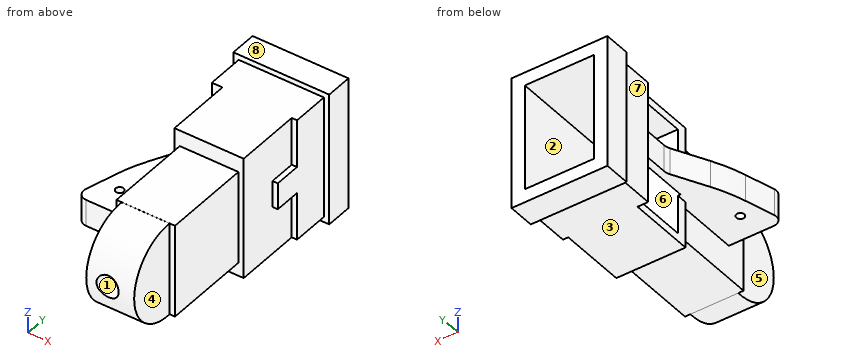
```python
from build123d import *

# Parameters (mm, degrees)
CONE002_ROLL_ANGLE   = 90
BOX005_W             = 26
BOX005_H             = 50
BOX005_DEPTH         = 40
BOX001_W             = 32
BOX001_H             = 17
BOX001_DEPTH         = 46
BOX002_W             = 26
BOX002_H             = 12
BOX002_DEPTH         = 10
BOX003_W             = 26
BOX003_H             = 26
BOX003_DEPTH         = 46
BOX004_W             = 22
BOX004_H             = 36
BOX004_DEPTH         = 35
CYLINDER_R           = 17.5
CYLINDER_DEPTH       = 18
CYLINDER_PITCH_ANGLE = 90
SKETCH001_R          = 1.5
PAD_DEPTH            = 4.5
PAD_DEPTH_BACK       = 5.5
BOX_W                = 36
BOX_H                = 10
BOX_DEPTH            = 50


with BuildPart() as obj1:
    # Cone002 → Cone002 (revolve)
    with BuildSketch(Plane.XZ):
        Polygon((0, 0), (3.9, 0), (4.2, 11), (0, 11), align=None)
    revolve(axis=Axis((0, 0, 0), (0, 0, 1)))


with BuildPart() as obj1_1:
    # Cone002 roll: moved
    add(obj1.part.rotate(Axis((0, 0, 0), (1, 0, 0)), CONE002_ROLL_ANGLE))


with BuildPart() as obj1_2:
    # Cone002 placement: moved
    add(obj1_1.part.moved(Location((32, 35, 35.5))))


with BuildPart() as kopfloch:
    # Box005 → Box005 (new body)
    with BuildSketch(Plane(origin=(19, 81, 16), x_dir=(1, 0, 0), z_dir=(0, 0, 1))):
        with Locations((13, 25)):
            Rectangle(BOX005_W, BOX005_H)
    extrude(amount=BOX005_DEPTH)


with BuildPart() as obj2:
    # Box001 → Box001 (new body)
    with BuildSketch(Plane(origin=(16, 102, 13), x_dir=(1, 0, 0), z_dir=(0, 0, 1))):
        with Locations((16, 8.5)):
            Rectangle(BOX001_W, BOX001_H)
    extrude(amount=BOX001_DEPTH)


with BuildPart() as obj3:
    # Box002 → Box002 (new body)
    with BuildSketch(Plane(origin=(22, 92, 31), x_dir=(1, 0, 0), z_dir=(0, 0, 1))):
        with Locations((13, 6)):
            Rectangle(BOX002_W, BOX002_H)
    extrude(amount=BOX002_DEPTH)


with BuildPart() as obj4:
    # Box003 → Box003 (new body)
    with BuildSketch(Plane(origin=(20, 77, 13), x_dir=(1, 0, 0), z_dir=(0, 0, 1))):
        with Locations((13, 13)):
            Rectangle(BOX003_W, BOX003_H)
    extrude(amount=BOX003_DEPTH)


with BuildPart() as obj5:
    # Box004 → Box004 (new body)
    with BuildSketch(Plane(origin=(22, 44, 18), x_dir=(1, 0, 0), z_dir=(0, 0, 1))):
        with Locations((11, 18)):
            Rectangle(BOX004_W, BOX004_H)
    extrude(amount=BOX004_DEPTH)


with BuildPart() as obj6:
    # Cylinder → Cylinder (new body)
    with BuildSketch(Plane.XY):
        Circle(CYLINDER_R)
    extrude(amount=CYLINDER_DEPTH)


with BuildPart() as obj6_1:
    # Cylinder pitch: moved
    add(obj6.part.rotate(Axis((0, 0, 0), (0, 1, 0)), CYLINDER_PITCH_ANGLE))


with BuildPart() as obj6_2:
    # Cylinder placement: moved
    add(obj6_1.part.moved(Location((24, 43, 35.5))))


with BuildPart() as obj7:
    # Sketch001 → Pad (new body, two sides)
    with BuildSketch(Plane(origin=(22, 44, 36), x_dir=(1, 0, 0), z_dir=(0, 0, 1))) as pad_sk:
        with BuildLine():
            Line((1.5, 7.670836), (-16.920451, 7.670836))
            ThreePointArc((-20.14616, 11.888508), (-19.57535, 8.982708), (-16.920451, 7.670836))
            Line((-20.14616, 11.888508), (-17.171201, 22.851854))
            ThreePointArc((-12.625578, 34.600006), (-15.204729, 28.844459), (-17.171201, 22.851854))
            Line((-12.625578, 34.600006), (-6.240143, 47.065773))
            ThreePointArc((-6.240143, 47.065773), (-5.840064, 48.144871), (-5.704179, 49.287696))
            Line((-5.704179, 49.287696), (-5.704179, 58.874008))
            Line((-5.704179, 58.874008), (1.5, 58.874008))
            Line((1.5, 58.874008), (1.5, 7.670836))
        make_face()
        with Locations((-11.5, 17.644535)):
            Circle(SKETCH001_R, mode=Mode.SUBTRACT)
    extrude(amount=PAD_DEPTH)
    extrude(pad_sk.sketch, amount=-PAD_DEPTH_BACK)


with BuildPart() as kopf:
    # Box → Box (new body)
    with BuildSketch(Plane(origin=(14, 116, 11), x_dir=(1, 0, 0), z_dir=(0, 0, 1))):
        with Locations((18, 5)):
            Rectangle(BOX_W, BOX_H)
    extrude(amount=BOX_DEPTH)

    # Fusion: union obj2, obj3, obj4, obj5, obj6, obj7
    add(obj2.part)
    add(obj3.part)
    add(obj4.part)
    add(obj5.part)
    add(obj6_2.part)
    add(obj7.part)

    # Cut: cut kopfloch
    add(kopfloch.part, mode=Mode.SUBTRACT)

    # Cut001: cut obj1
    add(obj1_2.part, mode=Mode.SUBTRACT)


solid = kopf.part
```
Source: CAD feature listing. Evaluate the final solid. Frame: model axes, mm. Face numbers are marked on the shaded views. A direction names the side the tool comes from. Round coordinates to 2 decimals unless told otherwise and drop trailing zeros. Write each loop counter-clockwise with the first axis right and the second up, starting at its lowest first coordinate (ties: lowest second). Pieces come first, ordered by that corner, then holes. Notation, with made-up numbers: M 85.5,57 L 98.5,57 A21 cw 98.5,74 Z; hole C 40,47.5 d9. An arc over 180 degrees is marked long. Answer as a JSON object with one key per item and string values. Group by question number.
(1) Reachability of the marked faces 1, 2, 3, 4 and 5 from +Z, -Z, +X, -X, +Y, -Y: full face, straight path, thin tool, end or side. Return the list, or none.
(2) Section query A-A on z = 54. Output: boundary loops of the cut face in (x, y), then the cut area to 3 significant figures.
(3) Section query C-C on x = 10.5. Output: boundary loops of the cut face in (y, z), then the cut area to 3 significant figures.
(4) Section query B-B on y = 119. Output: boundary loops of the cut face in (x, z).
(5) Mould query, pull axis Y, two halves, no side actions, for the marked faces 6, 7 and 8. Classes: +Y half, -Y half, draft (parallel to the pull), parting line (faces both ways), or undercut.
(6) First-contact query: pin 1 (17.5 mm diameter, centred on x = 28, y = 64.5, fed in from -Z); pin 2 (1 mm diameter, centred on x = 28.5, y = 63.5, fed in from +Z); pin 3 (16 mm diameter, centred on x = 37, y = 96, fed in from -Z). Flat tips, straight axial feed; report the tip coordinate or a pass-through.
(7) Ray query, line 1 (X direction, y = 119, z = 46); line 2 (X direction, y = 107, z = 38.5); line 3 (X direction, y = 71.5, z = 46). Return the intervals inside material, ascending. Write a range as [from, to].
(8) Section query D-D on z = 25. Output: boundary loops of the cut face in (x, y).
Computed values:
{
 "1": {"face 1": "-Y", "face 2": "+Y", "face 3": "-Z, +X, -X, -Y", "face 4": "+Z, -Z, +X, -Y", "face 5": "+Z, -Z, -X, -Y"},
 "2": {"outline": "M 14,116 L 16,116 L 16,102 L 19,102 L 19,126 L 14,126 Z; M 20,77 L 46,77 L 46,102 L 48,102 L 48,116 L 50,116 L 50,126 L 45,126 L 45,81 L 20,81 Z", "area": "309 mm^2"},
 "3": {"outline": "M 51.67,30.5 L 60.14,30.5 L 60.14,40.5 L 51.67,40.5 Z; M 63.14,30.5 L 80.8,30.5 L 80.8,40.5 L 63.14,40.5 Z", "area": "261 mm^2"},
 "4": {"outline": "M 14,11 L 50,11 L 50,61 L 14,61 Z; hole M 19,16 L 45,16 L 45,56 L 19,56 Z"},
 "5": {"face 6": "+Y half", "face 7": "undercut", "face 8": "draft"},
 "6": {"pin 1": "z = 18", "pin 2": "z = 53", "pin 3": "z = 13"},
 "7": {"line 1": "[14, 19], [45, 50]", "line 2": "[16, 19], [45, 48]", "line 3": "[22, 44]"},
 "8": {"outline": "M 14,116 L 16,116 L 16,102 L 19,102 L 19,126 L 14,126 Z; M 20,77 L 22,77 L 22,44 L 24,44 L 24,29 L 42,29 L 42,44 L 44,44 L 44,77 L 46,77 L 46,102 L 48,102 L 48,116 L 50,116 L 50,126 L 45,126 L 45,81 L 20,81 Z"}
}
